Work out the finished part from the listing and answer in its coordinate system (mm). Give positions to 0.01 mm unless a question says otherwise; leave off trailing zeros. Loops run counter-clockwise (first coordinate to the right, second up) from the corner with the lowest first, then second, coordinate; pieces in that order, holes last. Notation, with made-up numbers: (-12, -17.5) - (-7, -17.5) arc R17 ccw to (-7, 9.5) - close; hole circle Ø9 at (51.5, -39). An arc over 180 degrees is marked (long way). Use CSV: the item, a comma, the result in double quotes.
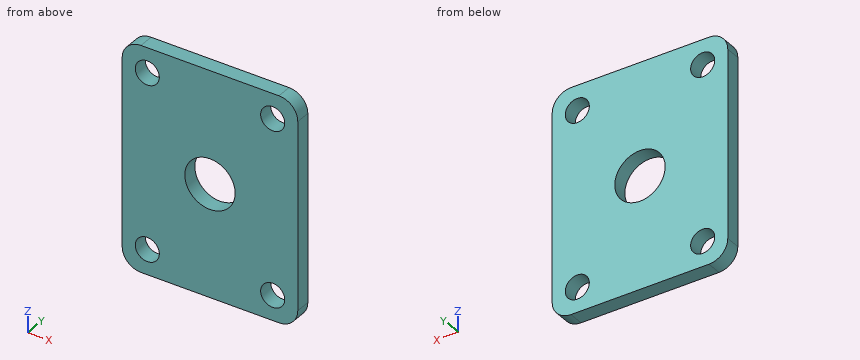
Autodesk Inventor part; units mm, degrees
ref_plane "YZ Plane" through (0, 0, 0) normal (1, 0, 0) x (0, 1, 0)
ref_plane "XZ Plane" through (0, 0, 0) normal (0, 1, 0) x (-1, 0, 0)
ref_plane "XY Plane" through (0, 0, 0) normal (0, 0, 1) x (1, 0, 0)
sketch "Sketch1" plane through (0, 0, 0) normal (0, 1, 0) x (-1, 0, 0)
  line L0 (0, -16.002) -> (0, 16.002)
  line L1 (-12.446, 0) -> (12.446, 0)
  line L2 (-8.89, 11.43) -> (8.89, 11.43)
  line L3 (8.89, 11.43) -> (8.89, -11.43)
  line L4 (8.89, -11.43) -> (-8.89, -11.43)
  line L5 (-8.89, -11.43) -> (-8.89, 11.43)
  line L6 (-8.89, 11.43) -> (8.89, -11.43) construction
  line L7 (8.89, 11.43) -> (-8.89, -11.43) construction
  point P0 (0, 0)
  point P1 (6.35, 8.89)
  point P2 (-6.35, 8.89)
  dimension "d0" = 6.35
  dimension "d1" = 6.35
  dimension "d23" = 22.86
  dimension "d24" = 17.78
  dimension "d25" = 8.89
extrude "Extrusion1" add sketch "Sketch1" against normal blind 1.524
hole "Hole1" at (-6.35, 0, 8.89) at (6.35, 0, 8.89) direction (0, -1, 0) diameter 2.4384 end through all
sketch "Sketch2" plane through (0, -1.524, 0) normal (0, -1, 0) x (1, 0, 0)
  line L0 (0, 16.002) -> (0, -16.002)
  line L1 (-12.446, 0) -> (12.446, 0)
  line L2 (-6.477, -4.064) -> (6.477, -4.064)
  line L3 (6.477, -4.064) -> (6.477, 4.064)
  line L4 (6.477, 4.064) -> (-6.477, 4.064)
  line L5 (-6.477, 4.064) -> (-6.477, -4.064)
  line L6 (-6.477, -4.064) -> (6.477, 4.064) construction
  line L7 (6.477, -4.064) -> (-6.477, 4.064) construction
  point P0 (0, 0)
  dimension "d11" = 12.954
  dimension "d12" = 8.128
extrude "Extrusion2" [suppressed]
hole "Hole2" at (0, 0, 0) direction (0, -1, 0) diameter 5.1054 end through all
fillet "Fillet1" radius 1.905 4 edges at (-8.89, -0.762, -11.43) (-8.89, -0.762, 11.43) (8.89, -0.762, 11.43) (8.89, -0.762, -11.43)
mirror "Mirror1" about plane through (0, 0, 0) normal (0, 0, 1) of "Hole1"
properties part number "J010354" material "STAINLESS STEEL, 304"
Item 1: A cutting plane is placed at C-C on y = -1.2. Determine the outline of the cut face in (x, z) (3 decimals).
Determined:
outline,"(-8.89, -9.525) arc R1.905 ccw to (-6.985, -11.43) - (6.985, -11.43) arc R1.905 ccw to (8.89, -9.525) - (8.89, 9.525) arc R1.905 ccw to (6.985, 11.43) - (-6.985, 11.43) arc R1.905 ccw to (-8.89, 9.525) - close; hole circle Ø2.438 at (-6.35, -8.89); hole circle Ø2.438 at (-6.35, 8.89); hole circle Ø5.105 at (0, 0); hole circle Ø2.438 at (6.35, -8.89); hole circle Ø2.438 at (6.35, 8.89)"
Item 2: Find the intervals of material crossed by line 1 (X direction, y = -0.8, z = -8.89); line 2 (Z direction, x = 6.35, y = -0.65); line 3 (Z direction, x = 5.25, y = -0.7), in increasing order.
Determined:
line 1,"x = -8.89 to -7.57, -5.13 to 5.13, 7.57 to 8.89"
line 2,"z = -11.43 to -10.11, -7.67 to 7.67, 10.11 to 11.43"
line 3,"z = -11.43 to -9.42, -8.36 to 8.36, 9.42 to 11.43"
Item 3: A cutting plane is placed at D-D on x = 0. Determine the outline of the cut face in (y, z), and give its area (3 significant figures).
Determined:
outline,"(-1.52, -11.43) - (0, -11.43) - (0, -2.55) - (-1.52, -2.55) - close; (-1.52, 2.55) - (0, 2.55) - (0, 11.43) - (-1.52, 11.43) - close"
area,"27.1 mm²"
Item 4: A cutting plane is placed at B-B on x = -6.35. Determine the outline of the cut face in (y, z).
Determined:
outline,"(-1.52, -11.43) - (0, -11.43) - (0, -10.11) - (-1.52, -10.11) - close; (-1.52, -7.67) - (0, -7.67) - (0, 7.67) - (-1.52, 7.67) - close; (-1.52, 10.11) - (0, 10.11) - (0, 11.43) - (-1.52, 11.43) - close"
Item 5: A cutting plane is placed at A-A on z = 0. Determine the outline of the cut face in (x, y), and give its area (3 significant figures).
Determined:
outline,"(-8.89, -1.52) - (-2.55, -1.52) - (-2.55, 0) - (-8.89, 0) - close; (2.55, -1.52) - (8.89, -1.52) - (8.89, 0) - (2.55, 0) - close"
area,"19.3 mm²"
